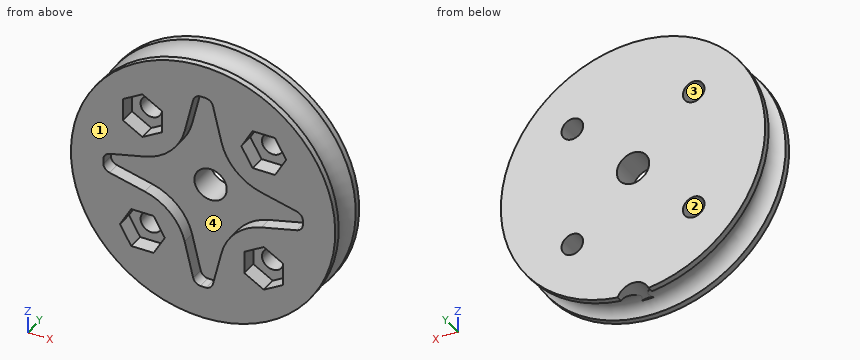
from build123d import *

# Parameters (mm, degrees)
CUT_EXTRUDE_1_DEPTH = 2.5
CUT_EXTRUDE_2_DEPTH = 3
SKETCH_6_R          = 2
CUT_EXTRUDE_4_DEPTH = 36.007142128
SKETCH_8_R          = 3.1
CUT_EXTRUDE_6_DEPTH = 5


with BuildPart() as part:
    # 草图2 → 旋转1 (revolve)
    with BuildSketch(Plane.XY, mode=Mode.PRIVATE) as revolve_1_sk:
        with BuildLine():
            Line((20, 8), (3, 8))
            Line((3, 8), (3, 0))
            Line((3, 0), (20, 0))
            Line((20, 0), (24.5, 0))
            Line((24.5, 0), (24.5, 1.06571985))
            Line((24.5, 1.06571985), (24.5, 1.145070053))
            ThreePointArc((24.5, 1.145070053), (22.475, 4), (24.5, 6.854929947))
            Line((24.5, 6.854929947), (24.5, 6.93428015))
            Line((24.5, 6.93428015), (24.5, 8))
            Line((24.5, 8), (20, 8))
        make_face()
    revolve(revolve_1_sk.sketch.rotate(Axis((0, 0, 0), (0, 1, 0)), 90), axis=Axis((0, 0, 0), (0, 1, 0)))

    # 草图3 → 切除-拉伸1 (cut)
    with BuildSketch(Plane.XZ):
        with BuildLine():
            Line((1.835992055, -17.350058041), (3.408354199, -10.798521635))
            ThreePointArc((3.408354199, -10.798521635), (6.061153739, -6.061181984), (10.798487471, -3.408371874))
            Line((10.798487471, -3.408371874), (17.350061912, -1.835985141))
            ThreePointArc((17.350061912, -1.835985141), (18.129967792, -1.363900547), (18.492480347, -0.527418811))
            Line((18.492480347, -0.527418811), (18.492480347, 0.527418811))
            ThreePointArc((18.492480347, 0.527418811), (18.129968102, 1.363905618), (17.350058041, 1.835992055))
            Line((17.350058041, 1.835992055), (10.798521635, 3.408354199))
            ThreePointArc((10.798521635, 3.408354199), (6.061181984, 6.061153739), (3.408371874, 10.798487471))
            Line((3.408371874, 10.798487471), (1.835985141, 17.350061912))
            ThreePointArc((1.835985141, 17.350061912), (1.363900547, 18.129967792), (0.527418811, 18.492480347))
            Line((0.527418811, 18.492480347), (-0.527418811, 18.492480347))
            ThreePointArc((-0.527418811, 18.492480347), (-1.363905618, 18.129968102), (-1.835992055, 17.350058041))
            Line((-1.835992055, 17.350058041), (-3.408354199, 10.798521635))
            ThreePointArc((-3.408354199, 10.798521635), (-6.061153739, 6.061181984), (-10.798487471, 3.408371874))
            Line((-10.798487471, 3.408371874), (-17.350061912, 1.835985141))
            ThreePointArc((-17.350061912, 1.835985141), (-18.129967792, 1.363900547), (-18.492480347, 0.527418811))
            Line((-18.492480347, 0.527418811), (-18.492480347, -0.527418811))
            ThreePointArc((-18.492480347, -0.527418811), (-18.129968102, -1.363905618), (-17.350058041, -1.835992055))
            Line((-17.350058041, -1.835992055), (-10.798521635, -3.408354199))
            ThreePointArc((-10.798521635, -3.408354199), (-6.061181984, -6.061153739), (-3.408371874, -10.798487471))
            Line((-3.408371874, -10.798487471), (-1.835985141, -17.350061912))
            ThreePointArc((-1.835985141, -17.350061912), (-1.363900547, -18.129967792), (-0.527418811, -18.492480347))
            Line((-0.527418811, -18.492480347), (0.527418811, -18.492480347))
            ThreePointArc((0.527418811, -18.492480347), (1.363905618, -18.129968102), (1.835992055, -17.350058041))
        make_face()
    extrude(amount=-CUT_EXTRUDE_1_DEPTH, mode=Mode.SUBTRACT)

    # 草图4 → 切除-拉伸2 (cut)
    with BuildSketch(Plane.XZ):
        Polygon((7.093078062, 11.25), (9.171539031, 7.65), (13.328460969, 7.65), (15.406921938, 11.25), (13.328460969, 14.85), (9.171539031, 14.85), align=None)
        Polygon((-11.25, 7.093078062), (-7.65, 9.171539031), (-7.65, 13.328460969), (-11.25, 15.406921938), (-14.85, 13.328460969), (-14.85, 9.171539031), align=None)
        Polygon((11.25, -7.093078062), (7.65, -9.171539031), (7.65, -13.328460969), (11.25, -15.406921938), (14.85, -13.328460969), (14.85, -9.171539031), align=None)
        Polygon((-7.093078062, -11.25), (-9.171539031, -7.65), (-13.328460969, -7.65), (-15.406921938, -11.25), (-13.328460969, -14.85), (-9.171539031, -14.85), align=None)
    extrude(amount=-CUT_EXTRUDE_2_DEPTH, mode=Mode.SUBTRACT)

    # 草图6 → 切除-拉伸4 (cut, through all)
    with BuildSketch(Plane.XZ.offset(-3)):
        with Locations(Location((-11.25, 11.25, 0), (0, 0, 270))):
            Circle(SKETCH_6_R)
        with Locations(Location((11.25, 11.25, 0), (0, 0, 270))):
            Circle(SKETCH_6_R)
        with Locations(Location((11.25, -11.25, 0), (0, 0, 270))):
            Circle(SKETCH_6_R)
        with Locations(Location((-11.25, -11.25, 0), (0, 0, 270))):
            Circle(SKETCH_6_R)
    extrude(amount=-CUT_EXTRUDE_4_DEPTH, mode=Mode.SUBTRACT)

    # 草图8 → 切除-拉伸6 (cut)
    with BuildSketch(Plane(origin=(0, 8, 0), x_dir=(1, 0, 0), z_dir=(0, 1, 0))):
        with Locations((0, 25.5)):
            Circle(SKETCH_8_R)
    extrude(amount=-CUT_EXTRUDE_6_DEPTH, mode=Mode.SUBTRACT)


solid = part.part
CAD build for the part. Positions are in the model's coordinates, mm. Face numbers are marked on the shaded views. A direction names the side the tool comes from. Round coordinates to 2 decimals unless told otherwise and drop trailing zeros. Write each question's results on one line, items separated by ' | '.
1. 3-axis set-ups, long thin cutter, end or side, ignore diameter. For the marked faces 3 and 4: which of +Z, -Z, +X, -X, +Y, -Y reach the whole face in a straight line?
Findings below:
face 3: +Y, -Y | face 4: -Y
2. Flat gauge pins, fed straight in: P1, Ø8, axis at x = 0, z = 0, coming from the -Y side; P2, Ø5, axis at x = 11.25, z = -11.25, coming from the -Y side; P3, Ø0.9, axis at y = 2, z = -10, coming from the +X side; P4, Ø3.5, axis at x = -11.25, z = -11.25, coming from the +Y side. Where does each tip first touch, or does it go through?
Findings below:
P1: stops at y = 2.5 | P2: stops at y = 3 | P3: stops at x = 21.55 | P4: passes through
3. Wall check: line 1 along X through (y, z) = (1.5, -14); line 2 along Z through (x, y) = (-10.5, 1); line 3 along X through (y, z) = (1.75, -15). Give the ranges that are in metal, low to high. Write a range as [from, to].
Findings below:
line 1: x = [-19.24, -13.82], [-8.68, -2.64], [2.64, 8.81], [13.69, 19.24] | line 2: z = [-22.14, -14.85], [-7.65, -3.48], [3.48, 7.53], [14.97, 22.14] | line 3: x = [-18.06, -2.4], [2.4, 10.55], [11.95, 18.06]
4. Pull direction Z, two halves, no side cores. Call the marked faces 1 and 2: pulls with the +Z half, pulls with the -Z half, needs draft (parallel to the pull), parting line crosses it, or undercut.
Findings below:
face 1: needs draft | face 2: undercut
